Check sheet for the modelled part. Datum: model origin and axes. Units: mm. Face numbers are marked on the shaded views. A direction names the side the tool comes from. Round coordinates to 2 decimals unless told otherwise and drop trailing zeros. Write each loop counter-clockwise with the first axis right and the second up, starting at its lowest first coordinate (ties: lowest second). Pieces come first, ordered by that corner, then holes.
Item 1: Depth check by flat-ended pin: pin 1 (0.8 mm diameter, centred on x = 0, z = 0, fed in from +Y); pin 2 (1.5 mm diameter, centred on x = 1.5, y = -3, fed in from +Z); pin 3 (1 mm diameter, centred on x = -3, y = -5.5, fed in from -Z). Enter the tip coordinate at first touch or a pass-through.
Item 2: Release check for a two-part mould opening along X. For the marked faces 1, 2 and 3 record: pulls with the +X half, pulls with the -X half, needs draft (parallel to the pull), parting line crosses it, or undercut.
Item 3: Section check B-B, the plane y = -7.25. Record the cut outline in (x, z).
Item 4: Material ranges on line 1 along X through (y, z) = (-2.25, 0); line 2 along X through (y, z) = (-6.25, 0); line 3 along Y through (x, z) = (1.5, -2), recorded low to high.
Item 5: Section check D-D, the plane y = -2.25. Record the cut outline in (x, z).
Item 6: Set-up check for the marked faces 4, 5 and 6: record each of +Z, -Z, +X, -X, +Y, -Y from which the full face is reachable in a straight line by a thin tool's end or side.
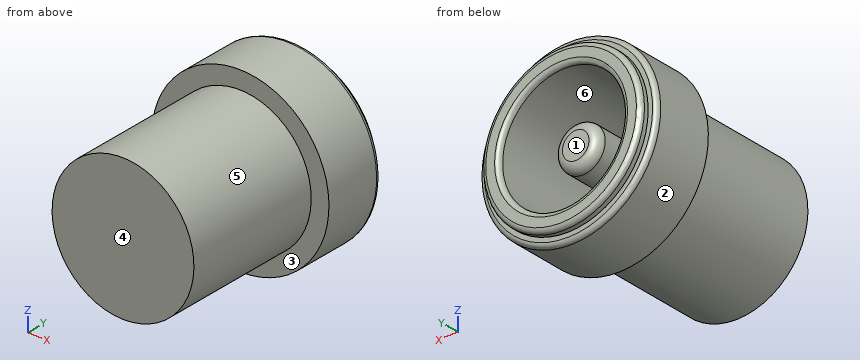
from build123d import *

# Parameters (mm, degrees)
SKETCH2_R            = 3.5
SKETCH2_R_2          = 1.25
INSIDE_CUT_DEPTH     = 10
SKETCH3_R            = 1.25
PIN_SHORTENING_DEPTH = 1
FILLET1_R            = 0.5
FILLET2_R            = 0.25


with BuildPart() as part:
    # Sketch1 → BULK (revolve)
    with BuildSketch(Plane.XY, mode=Mode.PRIVATE) as bulk_sk:
        Polygon((0, 0), (4.5, 0), (4.5, -0.5), (5, -0.5), (5, -4), (4, -4), (4, -12), (0, -12), align=None)
    revolve(bulk_sk.sketch.rotate(Axis((0, -12, 0), (0, 1, 0)), 90), axis=Axis((0, -12, 0), (0, 1, 0)))

    # Sketch2 → INSIDE CUT (cut)
    with BuildSketch(Plane(origin=(0, 0, 0), x_dir=(1, 0, 0), z_dir=(0, 1, 0))):
        with Locations(Location((0, 0, 0), (0, 0, 270))):
            Circle(SKETCH2_R)
        with Locations(Location((0, 0, 0), (0, 0, 270))):
            Circle(SKETCH2_R_2, mode=Mode.SUBTRACT)
    extrude(amount=-INSIDE_CUT_DEPTH, mode=Mode.SUBTRACT)

    # Sketch3 → PIN SHORTENING (cut)
    with BuildSketch(Plane(origin=(0, 0, 0), x_dir=(1, 0, 0), z_dir=(0, 1, 0))):
        with Locations(Location((0, 0, 0), (0, 0, 270))):
            Circle(SKETCH3_R)
    extrude(amount=-PIN_SHORTENING_DEPTH, mode=Mode.SUBTRACT)

    # Fillet1
    fillet1_edges = [part.edges().sort_by_distance(p)[0] for p in [
        (0, -1, -1.25),
    ]]
    fillet(fillet1_edges, radius=FILLET1_R)

    # Fillet2
    fillet2_edges = [part.edges().sort_by_distance(p)[0] for p in [
        (0, -10, -3.5),
        (0, 0, -3.5),
        (0, -0.5, 5),
        (0, 0, 4.5),
    ]]
    fillet(fillet2_edges, radius=FILLET2_R)


solid = part.part
Values found:
1. pin 1: stops at y = -1
1. pin 2: stops at z = 4.94
1. pin 3: stops at z = -3.12
2. face 1: undercut
2. face 2: parting line crosses it
2. face 3: needs draft
3. outline: circle Ø8 at (0, 0); circle Ø2.5 at (0, 0); hole circle Ø7 at (0, 0)
4. line 1: x = -5 to -3.5, -1.25 to 1.25, 3.5 to 5
4. line 2: x = -4 to -3.5, -1.25 to 1.25, 3.5 to 4
4. line 3: y = -12 to -10
5. outline: circle Ø10 at (0, 0); circle Ø2.5 at (0, 0); hole circle Ø7 at (0, 0)
6. face 4: +Z, -Z, +X, -X, -Y
6. face 5: -Y
6. face 6: +Y
